Geometry check sheet. Reference: the model listing, model coordinates, mm. Face numbers are marked on the shaded views. A direction names the side the tool comes from. Give positions to 0.01 mm unless a question says otherwise; leave off trailing zeros. Loops run counter-clockwise (first coordinate to the right, second up) from the corner with the lowest first, then second, coordinate; pieces in that order, holes last. Notation, with made-up numbers: (48, 2) -> (77, 2) arc R28 cw to (77, 21) -> close; hole circle Ø2 at (40.5, -38.75). An arc over 180 degrees is marked (long way). Answer as a JSON object with one key per item and string values.
from build123d import *

# Parameters (mm, degrees)
SKETCH_R          = 4
PAD_DEPTH         = 25
POCKET_DEPTH      = 70.001
POCKET_DEPTH_BACK = 10.001
PAD001_DEPTH      = 11.78


with BuildPart() as part:
    # Sketch → Pad (new body)
    with BuildSketch(Plane.XY):
        Polygon((40, 15), (40, -15), (40, -45), (25, -45), (25, -55), (-25, -55), (-25, -45), (-40, -45), (-40, -15), (-40, 15), (-25, 15), (-25, 25), (25, 25), (25, 15), align=None)
        with Locations((-25, 0)):
            Circle(SKETCH_R, mode=Mode.SUBTRACT)
        with Locations((25, 0)):
            Circle(SKETCH_R, mode=Mode.SUBTRACT)
        with Locations((-25, -30)):
            Circle(SKETCH_R, mode=Mode.SUBTRACT)
        with Locations((25, -30)):
            Circle(SKETCH_R, mode=Mode.SUBTRACT)
    extrude(amount=PAD_DEPTH)

    # Sketch001 → Pocket (cut, two sides)
    with BuildSketch(Plane(origin=(0, 15, 0), x_dir=(-1, 0, 0), z_dir=(0, 1, 0))) as pocket_sk:
        with BuildLine():
            ThreePointArc((9.5, 11.5), (0, 21), (-9.5, 11.5))
            Line((-9.5, 11.5), (-9.5, 0))
            Line((-9.5, 0), (0, 0))
            Line((0, 0), (9.5, 0))
            Line((9.5, 0), (9.5, 11.5))
        make_face()
        Polygon((-40, 5), (-35, 10), (-25, 10), (-25, 15), (-15, 25), (-40, 25), align=None)
        Polygon((40, 5), (35, 10), (25, 10), (25, 15), (15, 25), (40, 25), align=None)
    extrude(amount=-POCKET_DEPTH, mode=Mode.SUBTRACT)
    extrude(pocket_sk.sketch, amount=POCKET_DEPTH_BACK, mode=Mode.SUBTRACT)

    # Sketch002 → Pad001 (new body)
    with BuildSketch(Plane(origin=(0, 25, 0), x_dir=(-1, 0, 0), z_dir=(0, 1, 0))):
        with BuildLine():
            Line((-9.5, 0), (-6.5, 0))
            Line((-6.5, 0), (-6.5, 11.5))
            ThreePointArc((6.5, 11.5), (0, 18), (-6.5, 11.5))
            Line((6.5, 11.5), (6.5, 0))
            Line((6.5, 0), (9.5, 0))
            Line((9.5, 0), (9.5, 11.5))
            ThreePointArc((9.5, 11.5), (0, 21), (-9.5, 11.5))
            Line((-9.5, 11.5), (-9.5, 0))
        make_face()
    extrude(amount=-PAD001_DEPTH)


solid = part.part
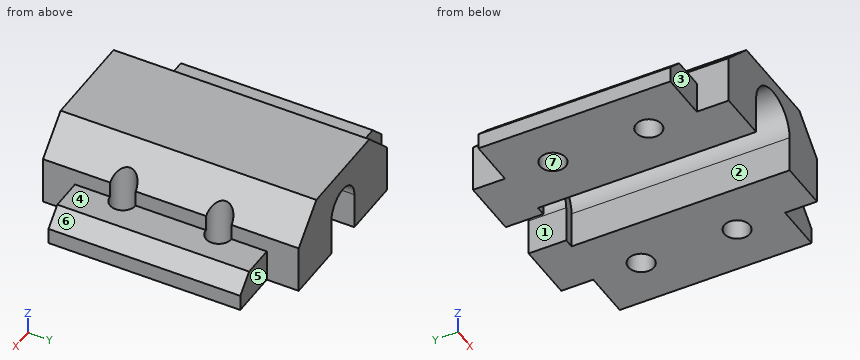
1) Section check B-B on y = 0. Record the cut outline in (x, z), plus the area to 3 significant figures.
Geometry check:
{"outline": "(-40, 0) -> (-29, 0) -> (-29, 10) -> (-35, 10) -> (-40, 5) -> close; (-21, 0) -> (-9.5, 0) -> (-9.5, 11.5) arc R9.5 cw to (9.5, 11.5) -> (9.5, 0) -> (21, 0) -> (21, 19) -> (15, 25) -> (-15, 25) -> (-21, 19) -> close; (29, 0) -> (40, 0) -> (40, 5) -> (35, 10) -> (29, 10) -> close", "area": "849 mm2"}
2) Tool access check on the marked faces 1, 2, 3 and 4. Record the directions out of +Z, -Z, +X, -X, +Y, -Y that give a thin tool (end or side, any length) a straight path to the whole face; none if there is none.
Geometry check:
{"face 1": "-Z, +Y, -Y", "face 2": "-Z, -Y", "face 3": "+Z, -Z, -X, -Y", "face 4": "+Z, +X, +Y, -Y"}
3) Depth check by flat-ended pin: P1, Ø6, axis at y = 19, z = 6.5, coming from the -X side; P2, Ø7, axis at x = 25, y = 0, coming from the +Z side; P3, Ø2, axis at y = -23.5, z = 6.5, coming from the -X side; P4, Ø6, axis at y = -11, z = 21, coming from the -X side. Enter the tip coordinate at first touch or a pass-through.
Geometry check:
{"P1": "stops at x = -25", "P2": "passes through", "P3": "stops at x = -39.5", "P4": "stops at x = -22"}
4) Material ranges on line 1 along X through (y, z) = (0, 4.25); line 2 along X through (y, z) = (0, 10.5); line 3 along X through (y, z) = (17.5, 5.75), recorded low to high. Write a range as from..to.
Geometry check:
{"line 1": "x = -40..-29, -21..-9.5, 9.5..21, 29..40", "line 2": "x = -21..-9.5, 9.5..21", "line 3": "x = -25..-6.5, 6.5..25"}
5) Section check A-A on z = 7.5. Record the cut outline in (x, y), plus the area to 3 significant figures.
Geometry check:
{"outline": "(-37.5, -45) -> (-25, -45) -> (-25, -55) -> (-9.5, -55) -> (-9.5, 13.22) -> (-6.5, 13.22) -> (-6.5, 25) -> (-25, 25) -> (-25, 15) -> (-37.5, 15) -> close; (6.5, 13.22) -> (9.5, 13.22) -> (9.5, -55) -> (25, -55) -> (25, -45) -> (37.5, -45) -> (37.5, 15) -> (25, 15) -> (25, 25) -> (6.5, 25) -> close; hole circle Ø8 at (-25, -30); hole circle Ø8 at (-25, 0); hole circle Ø8 at (25, -30); hole circle Ø8 at (25, 0)", "area": "3,850 mm2"}
6) Section check C-C on x = 0. Record the cut outline in (y, z), plus the area to 3 significant figures.
Geometry check:
{"outline": "(-55, 21) -> (13.22, 21) -> (13.22, 18) -> (25, 18) -> (25, 25) -> (-55, 25) -> close", "area": "355 mm2"}
7) Draft check along X on the marked faces 5, 6 and 7. Enter one of: pulls with the +X half, pulls with the -X half, needs draft (parallel to the pull), parting line crosses it, or undercut.
Geometry check:
{"face 5": "needs draft", "face 6": "pulls with the +X half", "face 7": "undercut"}
